```python
from build123d import *

# Parameters (mm, degrees)
SKETCH_1_W          = 96
SKETCH_1_H          = 20
EXTRUDE_1_DEPTH     = 82
CUT_EXTRUDE_2_DEPTH = 20
SKETCH_3_W          = 40
SKETCH_3_H          = 15.5
CUT_EXTRUDE_3_DEPTH = 76
SKETCH_6_R          = 1.5
CUT_EXTRUDE_5_DEPTH = 10


with BuildPart() as part:
    # 草图1 → 凸台-拉伸1 (new body)
    with BuildSketch(Plane.XY):
        with Locations((48, 10)):
            Rectangle(SKETCH_1_W, SKETCH_1_H)
    extrude(amount=EXTRUDE_1_DEPTH)

    # 草图2 → 切除-拉伸2 (cut)
    with BuildSketch(Plane(origin=(0, 20, 0), x_dir=(1, 0, 0), z_dir=(0, 1, 0))):
        with BuildLine():
            Line((17, -82), (35, -82))
            ThreePointArc((35, -82), (26, -73), (17, -82))
        make_face()
        with BuildLine():
            Line((79, -82), (61, -82))
            ThreePointArc((61, -82), (70, -73), (79, -82))
        make_face()
    extrude(amount=-CUT_EXTRUDE_2_DEPTH, mode=Mode.SUBTRACT)

    # 草图3 → 切除-拉伸3 (cut)
    with BuildSketch(Plane.XY.offset(82)):
        with Locations((26, 10.25)):
            Rectangle(SKETCH_3_W, SKETCH_3_H)
        with Locations((149, 10.25)):
            Rectangle(SKETCH_3_W, SKETCH_3_H)
        with Locations((70, 10.25)):
            Rectangle(SKETCH_3_W, SKETCH_3_H)
    extrude(amount=-CUT_EXTRUDE_3_DEPTH, mode=Mode.SUBTRACT)

    # 草图6 → 切除-拉伸5 (cut)
    with BuildSketch(Plane.XZ):
        with Locations(Location((86, 2.5, 0), (0, 0, 270))):
            Circle(SKETCH_6_R)
        with Locations(Location((10, 2.5, 0), (0, 0, 90))):
            Circle(SKETCH_6_R)
        with Locations(Location((93, 64, 0), (0, 0, 270))):
            Circle(SKETCH_6_R)
        with Locations(Location((3, 64, 0), (0, 0, 90))):
            Circle(SKETCH_6_R)
    extrude(amount=-CUT_EXTRUDE_5_DEPTH, mode=Mode.SUBTRACT)


solid = part.part
```
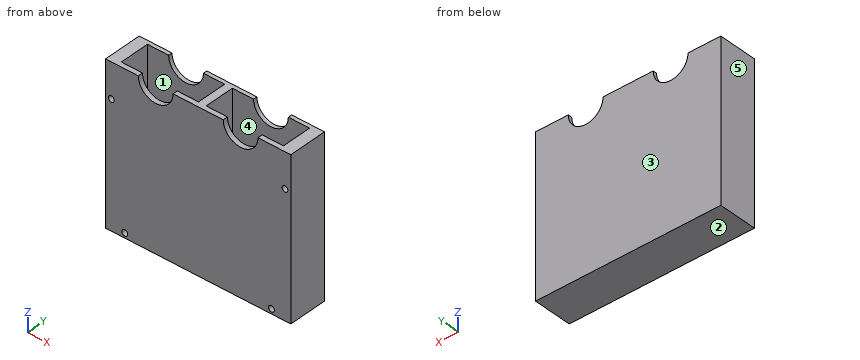
Design review of the part built by this model. Coordinates are the model's own, in mm. Face numbers are marked on the shaded views. A direction names the side the tool comes from. Give positions to 0.01 mm unless a question says otherwise; leave off trailing zeros. Write each loop counter-clockwise with the first axis right and the second up, starting at its lowest first coordinate (ties: lowest second). Pieces come first, ordered by that corner, then holes.
(1) Add section B-B (y = 7). Give the boundary of the cut face in (x, z), and give its area (3 significant figures).
Checked values:
outline: (0, 0) - (96, 0) - (96, 82) - (90, 82) - (90, 6) - (50, 6) - (50, 82) - (46, 82) - (46, 6) - (6, 6) - (6, 82) - (0, 82) - close; hole circle Ø3 at (3, 64); hole circle Ø3 at (10, 2.5); hole circle Ø3 at (86, 2.5); hole circle Ø3 at (93, 64)
area: 1,760 mm2
(2) Add section C-C (x = 14). Give the boundary of the cut face in (y, z), and give its area (3 significant figures).
Checked values:
outline: (0, 0) - (20, 0) - (20, 82) - (18, 82) - (18, 6) - (2.5, 6) - (2.5, 82) - (0, 82) - close
area: 462 mm2
(3) Add section D-D (z = 2.5). Give the boundary of the cut face in (x, y), and give its area (3 significant figures).
Checked values:
outline: (0, 0) - (8.5, 0) - (8.5, 10) - (11.5, 10) - (11.5, 0) - (84.5, 0) - (84.5, 10) - (87.5, 10) - (87.5, 0) - (96, 0) - (96, 20) - (0, 20) - close
area: 1,860 mm2
(4) Tool access review of the marked faces 1 and 2: name each direction out of +Z, -Z, +X, -X, +Y, -Y from which nothing blocks a thin tool from reaching the whole face with its end or side.
Checked values:
face 1: +Z
face 2: -Z, +X, -X, +Y, -Y
(5) Wall thickness on line 1 along X through (y, z) = (7.75, 14.5); line 2 along X through (y, z) = (5.75, 64); line 3 along X through (y, z) = (6.5, 2.5): over which ranges is each line inside the solid? List them lowest first.
Checked values:
line 1: x = 0 to 6, 46 to 50, 90 to 96
line 2: x = 0 to 1.5, 4.5 to 6, 46 to 50, 90 to 91.5, 94.5 to 96
line 3: x = 0 to 8.5, 11.5 to 84.5, 87.5 to 96
(6) Add section A-A (z = 22). Give the boundary of the cut face in (x, y).
Checked values:
outline: (0, 0) - (96, 0) - (96, 20) - (0, 20) - close; hole (6, 2.5) - (46, 2.5) - (46, 18) - (6, 18) - close; hole (50, 2.5) - (90, 2.5) - (90, 18) - (50, 18) - close
(7) Clearance check with flat-ended pins moving along their axes: pin 1 Ø8 at (x, y) = (63, 8.5) entering from +Z; pin 2 Ø1.5 at (x, z) = (10.5, 3) entering from -Y. State where each tip first meets the part, or that it passes through.
Checked values:
pin 1: stops at z = 6
pin 2: stops at y = 10
(8) Mouldability with a two-part tool opening along X and no side actions: class the marked faces 3, 4 and 5 as +X half, -X half, draft (parallel to the pull), parting line (faces both ways), or undercut.
Checked values:
face 3: draft
face 4: undercut
face 5: -X half
